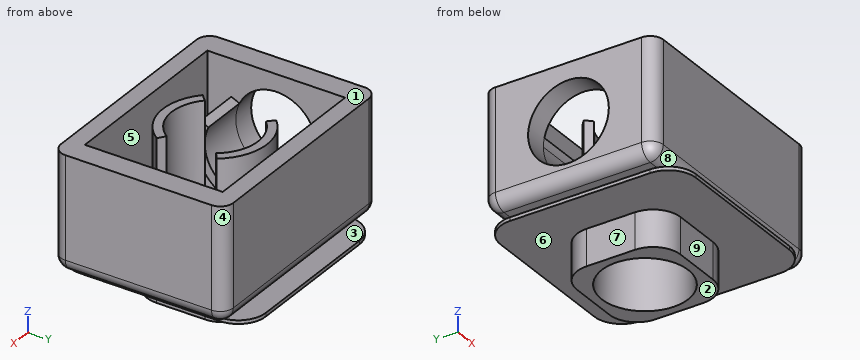
```python
from build123d import *

# Parameters (mm, degrees)
F0_W      = 50.8
F0_H      = 38.1
F1_DEPTH  = 25.4
F2_W      = 40.64
F2_H      = 30.48
F3_DEPTH  = 22.225
F4_R      = 9.5514218063
F5_DEPTH  = 25.4
F6_R      = 8.9260934587
F7_DEPTH  = 25.4
F9_DEPTH  = 10.3378
F11_DEPTH = 21.082
F12_W     = 22.86
F12_H     = 22.86
F12_R     = 10.7189198073
F12_R_2   = 9.5514218063
F13_DEPTH = 9.6266
F14_W     = 22.86
F14_H     = 0.79375
F15_DEPTH = 10.16
F17_DEPTH = 10.16
F18_W     = 10.16
F18_H     = 0.79375
F18_W_2   = 22.86
F19_DEPTH = 10.16
F20_W     = 10.16
F20_H     = 0.79375
F20_W_2   = 22.86
F21_DEPTH = 10.16
F22_R     = 6.0707814239
F23_R     = 2.8820881508


# Not quite as in the source:
# - a length typed as a fraction of an inch, garbled in the dataset ("3 / 203.2 mm" for 3/8 in), is restored
# - a feature names something its author has since deleted; it is built from what else it names


with BuildPart() as f1:
    # F0 (on Top) → F1 (new body)
    with BuildSketch(Plane.XY):
        with Locations((-32.453101594, -1.12241521)):
            Rectangle(F0_W, F0_H)
    extrude(amount=F1_DEPTH)

    # F2 (on face) → F3 (cut)
    with BuildSketch(Plane.XY.offset(25.4)):
        with Locations((-32.453101594, -1.12241521)):
            Rectangle(F2_W, F2_H)
    extrude(amount=-F3_DEPTH, mode=Mode.SUBTRACT)

    # F4 (on face) → F5 (cut)
    with BuildSketch(Plane.XY.offset(3.175)):
        with Locations((-32.453101594, -1.12241521)):
            Circle(F4_R)
    extrude(amount=-F5_DEPTH, mode=Mode.SUBTRACT)

    # F6 (on face) → F7 (cut)
    with BuildSketch(Plane(origin=(-57.853101594, 0, 0), x_dir=(0, -1, 0), z_dir=(-1, 0, 0))):
        with Locations((1.12241521, 12.7)):
            Circle(F6_R)
    extrude(amount=-F7_DEPTH, mode=Mode.SUBTRACT)

    # F8 (on face) → F9 (join)
    with BuildSketch(Plane.YZ.offset(-52.773101594)):
        with BuildLine():
            ThreePointArc((4.2283937472, 3.175), (8.3066529455, 7.1818974988), (9.8026377187, 12.7))
            ThreePointArc((9.8026377187, 12.7), (9.7389872891, 13.8775895924), (9.5487776675, 15.0414576799))
            Line((9.5487776675, 15.0414576799), (7.5962670299, 14.6130406248))
            ThreePointArc((7.5962670299, 14.6130406248), (7.7516739529, 13.6621257514), (7.8036782487, 12.7))
            ThreePointArc((7.8036782487, 12.7), (-3.0308273005, 3.9803034613), (-9.2324659679, 16.4285682425))
            Line((-9.2324659679, 16.4285682425), (-11.0486762552, 17.2635647427))
            ThreePointArc((-11.0486762552, 17.2635647427), (-11.5132347682, 9.3254407095), (-6.4732241672, 3.175))
            Line((-6.4732241672, 3.175), (4.2283937472, 3.175))
        make_face()
    extrude(amount=F9_DEPTH)

    # F10 (on face) → F11 (join)
    with BuildSketch(Plane.XY.offset(3.175)):
        with BuildLine():
            Line((-24.6290348955, 4.3560552717), (-23.0209375751, 5.4820571376))
            ThreePointArc((-23.0209375751, 5.4820571376), (-31.4495427718, 10.3483146168), (-40.5951152599, 7.0195984558))
            Line((-40.5951152599, 7.0195984558), (-39.2069767232, 5.6314599192))
            ThreePointArc((-39.2069767232, 5.6314599192), (-31.6206403322, 8.3926605526), (-24.6290348955, 4.3560552717))
        make_face()
        with BuildLine():
            ThreePointArc((-40.5951152599, -9.2644288759), (-31.4495427718, -12.5931450369), (-23.0209375751, -7.7268875577))
            Line((-23.0209375751, -7.7268875577), (-24.6290348955, -6.6008856918))
            ThreePointArc((-24.6290348955, -6.6008856918), (-31.6206403322, -10.6374909727), (-39.2069767232, -7.8762903393))
            Line((-39.2069767232, -7.8762903393), (-40.5951152599, -9.2644288759))
        make_face()
    extrude(amount=F11_DEPTH)

    # F12 (on face) → F13 (join)
    with BuildSketch(Plane(origin=(0, 0, 0), x_dir=(1, 0, 0), z_dir=(0, 0, -1))):
        with Locations((-32.453101594, 1.12241521)):
            Rectangle(F12_W, F12_H)
        with Locations((-32.453101594, 1.12241521)):
            Circle(F12_R, mode=Mode.SUBTRACT)
        with Locations((-32.453101594, 1.12241521)):
            Circle(F12_R)
        with Locations((-32.453101594, 1.12241521)):
            Circle(F12_R_2, mode=Mode.SUBTRACT)
    extrude(amount=F13_DEPTH)

    # F14 (on face) → F15 (join)
    with BuildSketch(Plane(origin=(0, 10.30758479, 0), x_dir=(-1, 0, 0), z_dir=(0, 1, 0))):
        with Locations((32.453101594, -1.190625)):
            Rectangle(F14_W, F14_H)
    extrude(amount=F15_DEPTH)

    # F16 (on face) → F17 (join)
    with BuildSketch(Plane.YZ.offset(-21.023101594)):
        Polygon((-12.55241521, -0.79375), (-12.55241521, -1.5875), (10.30758479, -1.5875), (20.46758479, -1.5875), (20.46758479, -0.79375), (10.30758479, -0.79375), align=None)
    extrude(amount=F17_DEPTH)

    # F18 (on face) → F19 (join)
    with BuildSketch(Plane.XZ.offset(12.55241521)):
        with Locations((-15.943101594, -1.190625)):
            Rectangle(F18_W, F18_H)
        with Locations((-32.453101594, -1.190625)):
            Rectangle(F18_W_2, F18_H)
    extrude(amount=F19_DEPTH)

    # F20 (on face) → F21 (join)
    with BuildSketch(Plane(origin=(-43.883101594, 0, 0), x_dir=(0, -1, 0), z_dir=(-1, 0, 0))):
        with Locations((-15.38758479, -1.190625)):
            Rectangle(F20_W, F20_H)
        with Locations((1.12241521, -1.190625)):
            Rectangle(F20_W_2, F20_H)
        with Locations((17.63241521, -1.190625)):
            Rectangle(F20_W, F20_H)
    extrude(amount=F21_DEPTH)

    # F22
    f22_edges = [f1.edges().sort_by_distance(p)[0] for p in [
        (-10.863102, 20.467585, -1.190625),
        (-54.043102, 20.467585, -1.190625),
        (-54.043102, -22.712415, -1.190625),
        (-10.863102, -22.712415, -1.190625),
        (-21.023102, -12.552415, -5.60705),
        (-43.883102, -12.552415, -5.60705),
        (-43.883102, 10.307585, -5.60705),
        (-21.023102, 10.307585, -5.60705),
    ]]
    fillet(f22_edges, radius=F22_R)

    # F23
    f23_edges = [f1.edges().sort_by_distance(p)[0] for p in [
        (-32.453102, -20.172415, 0),
        (-57.853102, -1.122415, 0),
        (-57.853102, -20.172415, 12.7),
        (-7.053102, -1.122415, 0),
        (-7.053102, -20.172415, 12.7),
        (-32.453102, 17.927585, 0),
        (-7.053102, 17.927585, 12.7),
        (-57.853102, 17.927585, 12.7),
    ]]
    fillet(f23_edges, radius=F23_R)


solid = f1.part
```
CAD build for the part. Positions are in the model's coordinates, mm. Face numbers are marked on the shaded views. A direction names the side the tool comes from. Give positions to 0.01 mm unless a question says otherwise; leave off trailing zeros. Order: outer loops, then holes, each group sorted by start corner. A loop starts at its lowest first (then second) coordinate and runs counter-clockwise, first axis right, second up.
(1) Saw through at A-A, the plane z = 23.5. Give the cut face in (x, y).
(2) Mould opens along Z. For the marked faces 1, 2, 3 and 4 say: released by +Z, released by -Z, zero draft, split by the parting line, or undercut.
(3) Saw through at B-B, the plane z = 8. Give the cut face in (x, y), then the cut area to 3 significant figures.
(4) Drill centre lines: L1, parallel to Y at x = -48, z = 17.5; L2, parallel to Z at x = -11.5, y = -10.5; L3, parallel to Z at x = -14.5, y = -1 (1 decimal). Where is each one in solid material? Low to high.
(5) Saw through at C-C, the plane y = -4. State how many separate pieces and enclosed holes the cut face has, then the cut area to 3 significant figures.
(6) Tool access for the marked faces 5, 6, 7, 8 and 9: list every direction of +Z, -Z, +X, -X, +Y, -Y with a clear straight run to the whole face (end or side of a thin tool).
(7) Flat gauge pins, fed straight in: pin 1 (1 mm diameter, centred on y = 2.5, z = 8.5, fed in from -X); pin 2 (2 mm diameter, centred on x = -20.5, z = 3.5, fed in from +Y); pin 3 (1.8 mm diameter, centred on x = -33.5, y = 8, fed in from +Z). Where does each tip first touch, or does it go through?
Results found:
1. outline: (-57.85, -17.29) arc R2.88 ccw to (-54.97, -20.17) - (-9.94, -20.17) arc R2.88 ccw to (-7.05, -17.29) - (-7.05, 15.05) arc R2.88 ccw to (-9.94, 17.93) - (-54.97, 17.93) arc R2.88 ccw to (-57.85, 15.05) - close; (-40.6, -9.26) arc R11.51 ccw to (-23.02, -7.73) - (-24.63, -6.6) arc R9.55 cw to (-39.21, -7.88) - close; (-40.6, 7.02) - (-39.21, 5.63) arc R9.55 cw to (-24.63, 4.36) - (-23.02, 5.48) arc R11.51 ccw to start; hole (-52.77, -16.36) - (-12.13, -16.36) - (-12.13, 14.12) - (-52.77, 14.12) - close
2. face 1: released by +Z
2. face 2: released by -Z
2. face 3: undercut
2. face 4: zero draft
3. outline: (-57.85, -17.29) arc R2.88 ccw to (-54.97, -20.17) - (-9.94, -20.17) arc R2.88 ccw to (-7.05, -17.29) - (-7.05, 15.05) arc R2.88 ccw to (-9.94, 17.93) - (-54.97, 17.93) arc R2.88 ccw to (-57.85, 15.05) - (-57.85, 6.47) - (-42.44, 6.47) - (-42.44, 8.74) - (-52.77, 8.74) - (-52.77, 14.12) - (-12.13, 14.12) - (-12.13, -16.36) - (-52.77, -16.36) - (-52.77, -10.98) - (-42.44, -10.98) - (-42.44, -8.71) - (-57.85, -8.71) - close; (-40.6, -9.26) arc R11.51 ccw to (-23.02, -7.73) - (-24.63, -6.6) arc R9.55 cw to (-39.21, -7.88) - close; (-40.6, 7.02) - (-39.21, 5.63) arc R9.55 cw to (-24.63, 4.36) - (-23.02, 5.48) arc R11.51 ccw to start
3. area: 732 mm2
4. L1: y = -20.17 to -16.36, 14.12 to 17.93
4. L2: z = -1.59 to -0.79, 0 to 25.4
4. L3: z = -1.6 to -0.8, 0 to 3.2
5. separate pieces: 3
5. enclosed holes: 0
5. area: 312 mm2
6. face 5: +Z
6. face 6: -Z
6. face 7: -Z, -X, +Y, -Y
6. face 8: +X, -X, -Y
6. face 9: -Z, +X, -X, -Y
7. pin 1: stops at x = -12.13
7. pin 2: stops at y = 17.93
7. pin 3: stops at z = 24.26
